Verification items for the finished model (mm, model axes). Face numbers are marked on the shaded views. A direction names the side the tool comes from. Give positions to 0.01 mm unless a question says otherwise; leave off trailing zeros. Order: outer loops, then holes, each group sorted by start corner. A loop starts at its lowest first (then second) coordinate and runs counter-clockwise, first axis right, second up. Notation, with made-up numbers: (-32.75, -21.5) - (-24.75, -21.5) arc R18 ccw to (-24.75, -6.5) - close; hole circle Ø7 at (-10.75, 30). An arc over 180 degrees is marked (long way). Answer as a JSON object with one key per item and string values. Group by question number.
(1) Mould release check, pull along X, two halves, no side actions. Record for the marked faces 4, 5, 6 and 7: +X half, -X half, draft (parallel to the pull), parting line (faces both ways), or undercut.
(2) Access from +Z, -Z, +X, -X, +Y, -Y to the whole of each face (thin tool, end or side, straight path). Record for the marked faces 1, 2 and 3.
(3) Depth check by flat-ended pin: pin 1 Ø12 at (y, z) = (-4, -11.5) entering from -X; pin 2 Ø4 at (x, y) = (-6, 1) entering from -Z; pin 3 Ø5 at (y, z) = (-0.5, -10) entering from -X; pin 4 Ø1 at (x, z) = (-5, 13) entering from +Y. Enter the tip coordinate at first touch or a pass-through.
(4) Section check A-A (x = 4.25). Record the boundary of the cut face in (y, z), then the cut area to 3 significant figures.
(5) Section check C-C (x = -2). Record the boundary of the cut face in (y, z).
(6) Section check B-B (z = 16). Record the boundary of the cut face in (x, y).
(7) Section check D-D (z = -16). Record the boundary of the cut face in (x, y).
(8) Thickness scan on line 1 (Y direction, x = -4.75, z = -16.5); line 2 (Z direction, x = 3, y = -1.75); line 3 (Z direction, x = 4.25, y = 11.25). Record the ranges inside material, lowest first.
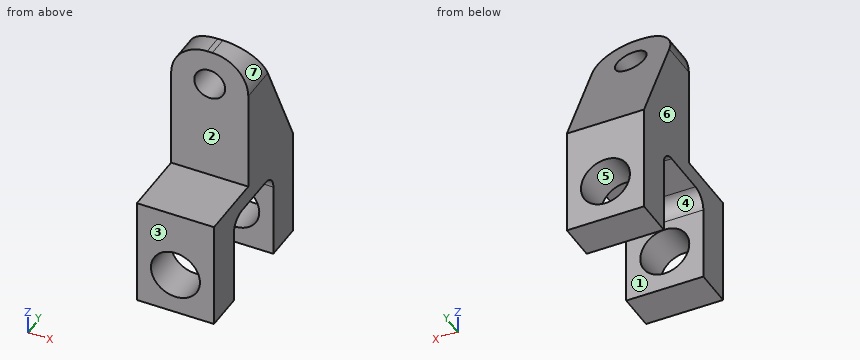
```python
from build123d import *

# Parameters (mm, degrees)
SKETCH1_W                = 15
SKETCH1_H                = 47.7777777
BOSS_EXTRUDE1_DEPTH      = 4
BOSS_EXTRUDE3_DEPTH      = 13
BOSS_EXTRUDE3_DEPTH_BACK = 17
SKETCH10_W               = 15
SKETCH10_H               = 21.082393169
SKETCH11_W               = 17.516789228
SKETCH11_H               = 15
CUT_EXTRUDE4_DEPTH       = 33.934465389
SKETCH12_R               = 4.765
CUT_EXTRUDE5_DEPTH       = 40.075939022
FILLET3_R                = 3
BOSS_EXTRUDE5_DEPTH      = 15
CUT_EXTRUDE7_DEPTH       = 31.264319098
CUT_EXTRUDE7_DEPTH_BACK  = 31.264319098
SKETCH3_R                = 3
FILLET4_R                = 7


with BuildPart() as part:
    # Sketch1 → Boss-Extrude1 (new body)
    with BuildSketch(Plane(origin=(0, 0, 0), x_dir=(1, 0, 0), z_dir=(0, 1, 0))):
        Rectangle(SKETCH1_W, SKETCH1_H)
    extrude(amount=BOSS_EXTRUDE1_DEPTH)

    # Sketch10 → Boss-Extrude3 (add, two sides: drawn at the far end of the back side and taken through both)
    with BuildSketch(Plane(origin=(0, 4, 0), x_dir=(1, 0, 0), z_dir=(0, 1, 0)).offset(-BOSS_EXTRUDE3_DEPTH_BACK)):
        with Locations((0, 13.347692266)):
            Rectangle(SKETCH10_W, SKETCH10_H)
    extrude(amount=BOSS_EXTRUDE3_DEPTH + BOSS_EXTRUDE3_DEPTH_BACK)

    # Sketch11 → Cut-Extrude4 (cut, through all)
    with BuildSketch(Plane(origin=(7.5, 0, 0), x_dir=(0, 0, -1), z_dir=(1, 0, 0))):
        with Locations((15.130494236, 2)):
            Rectangle(SKETCH11_W, SKETCH11_H)
    extrude(amount=-CUT_EXTRUDE4_DEPTH, mode=Mode.SUBTRACT)

    # Sketch12 → Cut-Extrude5 (cut, through all)
    with BuildSketch(Plane(origin=(0, 17, 0), x_dir=(1, 0, 0), z_dir=(0, 1, 0))):
        with Locations(Location((0, 15.806495681, 0), (0, 0, 270))):
            Circle(SKETCH12_R)
    extrude(amount=-CUT_EXTRUDE5_DEPTH, mode=Mode.SUBTRACT)

    # Fillet3
    fillet3_edges = [part.edges().sort_by_distance(p)[0] for p in [
        (0, -5.5, -6.372099622),
        (0, 9.5, -6.372099622),
    ]]
    fillet(fillet3_edges, radius=FILLET3_R)

    # Sketch14 → Boss-Extrude5 (add)
    with BuildSketch(Plane(origin=(7.5, 0, 0), x_dir=(0, 0, -1), z_dir=(1, 0, 0))):
        Polygon((2.806495681, 17), (-23.88888885, 4), (2.806495681, 4), align=None)
    extrude(amount=-BOSS_EXTRUDE5_DEPTH)

    # Sketch3 → Cut-Extrude7 (cut, two sides: drawn at the far end of the back side and taken through both)
    with BuildSketch(Plane(origin=(0, 4, 0), x_dir=(1, 0, 0), z_dir=(0, 1, 0)).offset(-CUT_EXTRUDE7_DEPTH_BACK)):
        with Locations(Location((0, -16.88888885, 0), (0, 0, 90))):
            Circle(SKETCH3_R)
    extrude(amount=CUT_EXTRUDE7_DEPTH + CUT_EXTRUDE7_DEPTH_BACK, mode=Mode.SUBTRACT)

    # Fillet4
    fillet4_edges = [part.edges().sort_by_distance(p)[0] for p in [
        (7.5, 2, 23.88888885),
        (-7.5, 2, 23.88888885),
    ]]
    fillet(fillet4_edges, radius=FILLET4_R)


solid = part.part
```
Solutions:
{
 "1": {"face 4": "draft", "face 5": "undercut", "face 6": "-X half", "face 7": "+X half"},
 "2": {"face 1": "-Z, +X, -X", "face 2": "+Z, +X, -X, -Y", "face 3": "+Z, -Z, +X, -X, -Y"},
 "3": {"pin 1": "stops at x = -7.5", "pin 2": "stops at z = -6.37", "pin 3": "passes through", "pin 4": "stops at y = 9.55"},
 "4": {"outline": "(-13, -23.89) - (-5.5, -23.89) - (-5.5, -17.96) - (-13, -17.96) - close; (-13, -13.65) - (-5.5, -13.65) - (-5.5, -9.37) arc R3 cw to (-2.5, -6.37) - (6.5, -6.37) arc R3 cw to (9.5, -9.37) - (9.5, -13.65) - (17, -13.65) - (17, -2.81) - (4.53, 22.8) - (0, 22.8) - (0, -2.81) - (-13, -2.81) - close; (9.5, -23.89) - (17, -23.89) - (17, -17.96) - (9.5, -17.96) - close", "area": "585 mm2"},
 "5": {"outline": "(-13, -23.89) - (-5.5, -23.89) - (-5.5, -20.13) - (-13, -20.13) - close; (-13, -11.48) - (-5.5, -11.48) - (-5.5, -9.37) arc R3 cw to (-2.5, -6.37) - (6.5, -6.37) arc R3 cw to (9.5, -9.37) - (9.5, -11.48) - (17, -11.48) - (17, -2.81) - (8.5, 14.65) - (0, 14.65) - (0, -2.81) - (-13, -2.81) - close; (0, 19.12) - (6.32, 19.12) - (4.08, 23.73) - (0, 23.73) - close; (9.5, -23.89) - (17, -23.89) - (17, -20.13) - (9.5, -20.13) - close"},
 "6": {"outline": "(-7.5, 0) - (-2.87, 0) - (-2.87, 7.84) - (-7.5, 7.84) - close; (2.87, 0) - (7.5, 0) - (7.5, 7.84) - (2.87, 7.84) - close"},
 "7": {"outline": "(-7.5, -13) - (-4.76, -13) - (-4.76, -5.5) - (-7.5, -5.5) - close; (-7.5, 9.5) - (-4.76, 9.5) - (-4.76, 17) - (-7.5, 17) - close; (4.76, -13) - (7.5, -13) - (7.5, -5.5) - (4.76, -5.5) - close; (4.76, 9.5) - (7.5, 9.5) - (7.5, 17) - (4.76, 17) - close"},
 "8": {"line 1": "y = -13 to -5.5, 9.5 to 17", "line 2": "z = -6.37 to -2.81", "line 3": "z = -23.89 to -17.96, -13.65 to 9"}
}
